```python
from build123d import *

# Parameters (mm, degrees)
F0_W     = 13.25
F0_H     = 65
F0_W_2   = 7.85
F0_H_2   = 14
F1_DEPTH = 2
F3_W     = 4.25
F3_H     = 2.1652186014
F4_DEPTH = 25
F5_R     = 0.5
F6_R     = 0.5
F7_R     = 0.2
F8_R     = 0.5


# Not quite as in the source:
# - the program builds the solid bodies; features that only make, move or delete a surface that nothing else refers to are left out


with BuildPart() as f1:
    # F0 (on Front) → F1 (new body)
    with BuildSketch(Plane.XZ):
        Rectangle(F0_W, F0_H)
        with Locations((0, 21.5)):
            Rectangle(F0_W_2, F0_H_2, mode=Mode.SUBTRACT)
    extrude(amount=F1_DEPTH)

    # F3 (on Front) → F4 (cut)
    with BuildSketch(Plane.XZ):
        with Locations((0, 32.5826093007)):
            Rectangle(F3_W, F3_H)
    extrude(amount=F4_DEPTH, mode=Mode.SUBTRACT)

    # F5
    f5_edges = [f1.edges().sort_by_distance(p)[0] for p in [
        (-2.125, -1, 32.5),
        (-6.625, -1, 32.5),
    ]]
    fillet(f5_edges, radius=F5_R)

    # F6
    f6_edges = [f1.edges().sort_by_distance(p)[0] for p in [
        (2.125, -1, 32.5),
        (6.625, -1, 32.5),
    ]]
    fillet(f6_edges, radius=F6_R)

    # F7
    f7_edges = [f1.edges().sort_by_distance(p)[0] for p in [
        (-3.925, -2, 21.5),
        (3.925, -2, 21.5),
        (3.925, 0, 21.5),
        (-3.925, 0, 21.5),
        (0, 0, 28.5),
        (0, -2, 28.5),
        (0, -2, 14.5),
        (0, 0, 14.5),
    ]]
    fillet(f7_edges, radius=F7_R)

    # F8
    f8_edges = [f1.edges().sort_by_distance(p)[0] for p in [
        (-6.625, 0, -0.25),
        (6.625, 0, -0.25),
    ]]
    fillet(f8_edges, radius=F8_R)


solid = f1.part
```
Model file for the job. Use its own axes, mm. A direction names the side the tool comes from. Coordinates: 2 decimals unless noted, no trailing zeros. Loops run counter-clockwise (first coordinate to the right, second up) from the corner with the lowest first, then second, coordinate; pieces in that order, holes last. Notation, with made-up numbers: (85.25, -2.5) - (90.25, -2.5) arc R14 ccw to (90.25, 3.5) - close; hole circle Ø1 at (49.5, 68). An arc over 180 degrees is marked (long way). Answer as a JSON object with one key per item and string values. Group by question number.
(1) Tool access for faces 4 (the face through (0, -1, 28.5)), 5 (the face through (6.625, -1, -1)): list every direction of +Z, -Z, +X, -X, +Y, -Y with a clear straight run to the whole face (end or side of a thin tool).
(2) Probe line 1 along Z through (x, y) = (-3.25, -0.5); line 2 along X through (y, z) = (-1, 24.5) (3 decimals); line 3 along Z through (x, y) = (-2, -0.9). List the from-to ranges inside material, lowest first.
(3) Cut at B-B (z = 27). Give the cut face in (x, y) (3 decimals).
(4) Cut at C-C (y = -1). Give the cut face in (x, z) (3 decimals).
(5) Two-plate mould, pull along Z, no slides. Class faces 1 (the face through (0, -1, 31.5)), 2 (the face through (3.925, -1, 21)), 3 (the face through (0, -2, 0)): released by +Z, released by -Z, zero draft, split by the parting line, or undercut.
(6) Cut at A-A (x = 0.75). Give the cut face in (y, z), then the cut area to 4 significant figures.
(7) Flat gauge pin, fed straight in: pin 1 (1 mm diameter, centred on x = 1, y = -1.5, fed in from +Z). Where does the tip first touch, or does it go through?
Geometry says:
{
 "1": {"face 4": "+Y, -Y", "face 5": "+Z, -Z, +X, +Y, -Y"},
 "2": {"line 1": "z = -32.5 to 14.5, 28.5 to 32.5", "line 2": "x = -6.625 to -3.925, 3.925 to 6.625", "line 3": "z = -32.5 to 14.5, 28.5 to 31.5"},
 "3": {"outline": "(-6.625, -2) - (-4.125, -2) arc R0.2 ccw to (-3.925, -1.8) - (-3.925, -0.2) arc R0.2 ccw to (-4.125, 0) - (-6.125, 0) arc R0.5 ccw to (-6.625, -0.5) - close; (3.925, -1.8) arc R0.2 ccw to (4.125, -2) - (6.625, -2) - (6.625, -0.5) arc R0.5 ccw to (6.125, 0) - (4.125, 0) arc R0.2 ccw to (3.925, -0.2) - close"},
 "4": {"outline": "(-6.625, -32.5) - (6.625, -32.5) - (6.625, 32) arc R0.5 ccw to (6.125, 32.5) - (2.625, 32.5) arc R0.5 ccw to (2.125, 32) - (2.125, 31.5) - (-2.125, 31.5) - (-2.125, 32) arc R0.5 ccw to (-2.625, 32.5) - (-6.125, 32.5) arc R0.5 ccw to (-6.625, 32) - close; hole (-3.925, 14.5) - (3.925, 14.5) - (3.925, 28.5) - (-3.925, 28.5) - close"},
 "5": {"face 1": "released by +Z", "face 2": "undercut", "face 3": "zero draft"},
 "6": {"outline": "(-2, -32.5) - (0, -32.5) - (0, 14.3) arc R0.2 ccw to (-0.2, 14.5) - (-1.8, 14.5) arc R0.2 ccw to (-2, 14.3) - close; (-2, 28.7) arc R0.2 ccw to (-1.8, 28.5) - (-0.2, 28.5) arc R0.2 ccw to (0, 28.7) - (0, 31.5) - (-2, 31.5) - close", "area": "100.0 mm^2"},
 "7": {"pin 1": "stops at z = 31.5"}
}
